Autodesk Inventor part; units mm, degrees
ref_plane "YZ Plane" through (0, 0, 0) normal (1, 0, 0) x (0, 1, 0)
ref_plane "XZ Plane" through (0, 0, 0) normal (0, 1, 0) x (-1, 0, 0)
ref_plane "XY Plane" through (0, 0, 0) normal (0, 0, 1) x (1, 0, 0)
sketch "Sketch2" plane through (0, 0, 0) normal (0, 0, 1) x (1, 0, 0)
  spline S0 degree 5 number of poles 204
  circle A0 centre (79.5137, 4.5678) radius 15.1135
  line L0 (79.5137, 4.5678) -> (79.5137, -15.4763) construction
  line L1 (79.5137, 4.5678) -> (209.6498, 4.5678) construction
  line L2 (319.6498, 0.0573) -> (219.6498, 0.0573) construction
  line L3 (219.6499, 18.7671) -> (219.6499, 18.7671) construction
  line L4 (28.0055, 4.5054) -> (28.0055, -2.4946)
  line L5 (19.6272, 1.0326) -> (319.6498, 0.0573) construction
  line L6 (49.7105, 14.4213) -> (55.6079, 14.4213)
  line L7 (49.7104, -8.4915) -> (55.6078, -8.4915)
  line L8 (28.0055, 4.5054) -> (49.7105, 14.4213)
  line L9 (28.0055, -2.4946) -> (49.7104, -8.4915)
  line L10 (55.6079, 14.4213) -> (55.6079, 20.8729)
  line L11 (55.6078, -8.4915) -> (55.6078, -14.1513)
  line L12 (108.6496, 16.3299) -> (108.6496, -7.1942)
  line L13 (110.8735, -9.1817) -> (193.8736, 0.1678)
  line L14 (195.6498, 2.1552) -> (195.6498, 6.9805)
  arc A1 (108.6496, -7.1942) -> (110.8735, -9.1817) centre (110.6496, -7.1942) ccw
  arc A2 (193.8736, 0.1678) -> (195.6498, 2.1552) centre (193.6498, 2.1552) ccw
  circle A3 centre (209.6498, 0.0573) radius 6.214
  line L15 (108.6496, 18.5678) -> (195.6498, 8.7678)
  circle A4 centre (100.6496, 18.3866) radius 2.5
  circle A5 centre (199.6498, 14.5256) radius 2.5
  spline S1 degree 4 poles (202.7347, 19.3724) (199.838, 19.7251) (195.7649, 20.2061) (190.5032, 20.7952) (184.0435, 21.4697) (179.3239, 21.937) (174.5933, 22.3806) (169.8562, 22.7962) (165.1183, 23.1863) (160.3828, 23.5463) (155.6566, 23.8767) (150.936, 24.1762) (146.2498, 24.4444) (141.5311, 24.676) (136.9019, 24.8782) (132.2312, 25.0296) (127.6189, 25.1375) (123.0371, 25.1983) (118.5028, 25.2125) (112.3622, 25.1677) (107.3995, 25.0507) (103.5849, 24.9119) (100.8865, 24.7866) knots 0 0 0 0 0 0.114234 0.16008 0.206003 0.251978 0.297982 0.343994 0.389991 0.435949 0.481846 0.527693 0.573431 0.619092 0.664656 0.710064 0.755333 0.800383 0.845191 0.889734 1 1 1 1 1
  line L16 (105.191, 21.4637) -> (195.6498, 15.3862)
  arc A6 (100.8865, 24.7866) -> (105.191, 21.4637) centre (100.0416, 19.2427) ccw
  arc A7 (195.6498, 15.3862) -> (202.7347, 19.3724) centre (200.4212, 15.1951) ccw
  point P0 (0, 0)
  point P1 (319.5771, 0.0748)
  point P2 (319.3573, 0.1272)
  point P3 (318.9916, 0.2136)
  point P4 (318.4804, 0.3362)
  point P5 (317.8238, 0.4909)
  point P6 (317.0222, 0.6802)
  point P7 (316.0769, 0.9024)
  point P8 (314.9885, 1.1569)
  point P9 (313.7582, 1.443)
  point P10 (312.3866, 1.7598)
  point P11 (310.8752, 2.1063)
  point P12 (309.2258, 2.4819)
  point P13 (307.4393, 2.8854)
  point P14 (305.5178, 3.3153)
  point P15 (303.4628, 3.7707)
  point P16 (301.2764, 4.2501)
  point P17 (298.9607, 4.7526)
  point P18 (296.5175, 5.2764)
  point P19 (293.9492, 5.8203)
  point P20 (291.2585, 6.3828)
  point P21 (288.4478, 6.9627)
  point P22 (285.5195, 7.5582)
  point P23 (282.4766, 8.1678)
  point P24 (279.3218, 8.79)
  point P25 (276.0584, 9.4236)
  point P26 (272.6891, 10.0668)
  point P27 (269.2175, 10.7178)
  point P28 (265.6469, 11.3757)
  point P29 (261.9803, 12.0381)
  point P30 (258.2219, 12.7041)
  point P31 (254.3747, 13.3722)
  point P32 (250.4426, 14.0403)
  point P33 (246.4295, 14.7072)
  point P34 (242.339, 15.3714)
  point P35 (238.1756, 16.0311)
  point P36 (233.9428, 16.6851)
  point P37 (229.6454, 17.3316)
  point P38 (225.2869, 17.9694)
  point P39 (220.8723, 18.5967)
  point P40 (216.4049, 19.2123)
  point P41 (211.8901, 19.8144)
  point P42 (207.332, 20.4015)
  point P43 (202.7347, 20.9724)
  point P44 (198.1034, 21.5256)
  point P45 (193.4423, 22.0596)
  point P46 (188.7563, 22.5726)
  point P47 (184.0499, 23.0637)
  point P48 (179.3279, 23.5314)
  point P49 (174.5948, 23.9745)
  point P50 (169.8554, 24.3909)
  point P51 (165.1148, 24.7803)
  point P52 (160.3775, 25.1406)
  point P53 (155.6479, 25.4709)
  point P54 (150.9316, 25.7703)
  point P55 (146.233, 26.0373)
  point P56 (141.557, 26.2707)
  point P57 (136.8821, 26.4681)
  point P58 (132.2209, 26.6211)
  point P59 (127.5964, 26.7282)
  point P60 (123.0133, 26.7888)
  point P61 (118.4727, 26.8026)
  point P62 (113.9902, 26.7693)
  point P63 (109.5601, 26.6886)
  point P64 (105.191, 26.5611)
  point P65 (100.8865, 26.3866)
  point P66 (96.6524, 26.1647)
  point P67 (92.4927, 25.8975)
  point P68 (88.412, 25.5858)
  point P69 (84.409, 25.3061)
  point P70 (80.8803, 24.9766)
  point P71 (76.6761, 24.4558)
  point P72 (72.9631, 23.8932)
  point P73 (69.3402, 23.3612)
  point P74 (65.8208, 22.7938)
  point P75 (62.4086, 22.1884)
  point P76 (59.1071, 21.5462)
  point P77 (52.8493, 20.1606)
  point P78 (49.7107, 19.4213)
  point P79 (47.0737, 18.6508)
  point P80 (44.3741, 17.8542)
  point P81 (41.8033, 17.0323)
  point P82 (39.3638, 16.1875)
  point P83 (37.0582, 15.3214)
  point P84 (34.8883, 14.4364)
  point P85 (32.8567, 13.534)
  point P86 (30.9649, 12.6166)
  point P87 (29.2144, 11.686)
  point P88 (27.607, 10.7437)
  point P89 (26.1442, 9.7921)
  point P90 (24.8269, 8.8324)
  point P91 (23.6566, 7.8664)
  point P92 (22.6337, 6.8952)
  point P93 (21.7592, 5.9208)
  point P94 (21.0335, 4.944)
  point P95 (20.4573, 3.966)
  point P96 (20.031, 2.9874)
  point P97 (19.7541, 2.0097)
  point P98 (19.6496, 0.0598)
  point P99 (19.8207, -0.9032)
  point P100 (20.1378, -1.8356)
  point P101 (20.6004, -2.7401)
  point P102 (21.2081, -3.6158)
  point P103 (21.9599, -4.4627)
  point P104 (22.8545, -5.2806)
  point P105 (23.891, -6.069)
  point P106 (25.0682, -6.8277)
  point P107 (26.3845, -7.5561)
  point P108 (27.8383, -8.2539)
  point P109 (29.4283, -8.9211)
  point P110 (31.1522, -9.5571)
  point P111 (33.0086, -10.1613)
  point P112 (34.9949, -10.734)
  point P113 (37.1093, -11.2746)
  point P114 (39.3497, -11.7828)
  point P115 (41.7134, -12.2586)
  point P116 (44.1979, -12.702)
  point P117 (46.8014, -13.1127)
  point P118 (49.7105, -13.4915)
  point P119 (52.3532, -13.8357)
  point P120 (58.3469, -14.4294)
  point P121 (61.5023, -14.678)
  point P122 (64.7591, -14.8953)
  point P123 (68.1149, -15.0813)
  point P124 (71.5661, -15.237)
  point P125 (75.1094, -15.3627)
  point P126 (78.7418, -15.4596)
  point P127 (82.46, -15.528)
  point P128 (86.2607, -15.5691)
  point P129 (90.14, -15.5838)
  point P130 (94.0946, -15.5733)
  point P131 (98.1212, -15.5388)
  point P132 (102.2159, -15.4812)
  point P133 (106.3751, -15.4023)
  point P134 (110.5952, -15.303)
  point P135 (114.872, -15.1845)
  point P136 (119.2022, -15.0489)
  point P137 (123.5813, -14.8971)
  point P138 (128.006, -14.7306)
  point P139 (132.4718, -14.5509)
  point P140 (136.9748, -14.3598)
  point P141 (141.5285, -14.1576)
  point P142 (146.1365, -13.9383)
  point P143 (150.7679, -13.7022)
  point P144 (155.4191, -13.4499)
  point P145 (160.0853, -13.1829)
  point P146 (164.7617, -12.9024)
  point P147 (169.4444, -12.6099)
  point P148 (174.1283, -12.306)
  point P149 (178.8092, -11.9925)
  point P150 (183.4823, -11.67)
  point P151 (188.1434, -11.34)
  point P152 (192.7877, -11.0037)
  point P153 (197.4107, -10.6614)
  point P154 (202.0079, -10.3149)
  point P155 (206.5747, -9.9645)
  point P156 (211.1069, -9.6117)
  point P157 (215.5999, -9.2568)
  point P158 (220.0489, -8.9007)
  point P159 (224.4503, -8.5446)
  point P160 (228.7987, -8.1885)
  point P161 (233.0906, -7.8339)
  point P162 (237.3214, -7.4808)
  point P163 (241.4866, -7.1298)
  point P164 (245.5828, -6.7821)
  point P165 (249.6052, -6.4377)
  point P166 (253.5502, -6.0972)
  point P167 (257.4136, -5.7612)
  point P168 (261.1915, -5.4303)
  point P169 (264.88, -5.1051)
  point P170 (268.4758, -4.7856)
  point P171 (271.9747, -4.4724)
  point P172 (275.3734, -4.1661)
  point P173 (278.6686, -3.867)
  point P174 (281.8564, -3.5757)
  point P175 (284.9344, -3.2925)
  point P176 (287.8984, -3.018)
  point P177 (290.7463, -2.7525)
  point P178 (293.4745, -2.4963)
  point P179 (296.0806, -2.2503)
  point P180 (298.5616, -2.0142)
  point P181 (300.9151, -1.7892)
  point P182 (303.1387, -1.575)
  point P183 (305.23, -1.3728)
  point P184 (307.1866, -1.1823)
  point P185 (309.007, -1.0041)
  point P186 (310.6885, -0.8385)
  point P187 (312.2302, -0.6861)
  point P188 (313.6297, -0.5471)
  point P189 (314.8861, -0.4221)
  point P190 (315.9976, -0.3107)
  point P191 (316.9636, -0.214)
  point P192 (317.7826, -0.1311)
  point P193 (318.4538, -0.0643)
  point P194 (318.9765, -0.0102)
  point P195 (319.3503, 0.027)
  point P196 (319.5743, 0.0497)
  point P197 (28.0055, 1.0054)
  point P198 (108.6496, -9.4322)
  point P199 (195.6498, 0.3678)
  dimension "d37" = 30.227
  dimension "d2" = 300.0001
  dimension "d19" = 110
  dimension "d22" = 100
  dimension "d23" = 7
  dimension "d24" = 5
  dimension "d25" = 5
  dimension "d30" = 28
  dimension "d31" = 8.4
  dimension "d33" = 14
  dimension "d39" = 59.8865
  dimension "d42" = 12.428
  dimension "d43" = 5
  dimension "d44" = 5
  dimension "d49" = 1.6
  dimension "d50" = 1.6
  dimension "d51" = 1.6
  dimension "d52" = 1.6
  dimension "d53" = 1.6
  dimension "d54" = 1.6
  dimension "d55" = 1.6
  dimension "d56" = 1.6
  dimension "d57" = 1.6
  dimension "d58" = 1.6
  dimension "d59" = 1.6
  dimension "d60" = 1.6
  dimension "d61" = 1.6
  dimension "d62" = 1.6
  dimension "d63" = 1.6
  dimension "d64" = 1.6
  dimension "d65" = 1.6
  dimension "d66" = 1.6
  dimension "d67" = 1.6
  dimension "d68" = 1.6
  dimension "d69" = 1.6
  dimension "d70" = 1.6
  dimension "d72" = 1.6
  dimension "d75" = 4
  dimension "d76" = 7
  dimension "d90" = 8
  dimension "d91" = 8
extrude "Extrusion8" add sketch "Sketch2" along normal blind 54 contours A7 L16 A6 S1
sketch "Sketch3" plane through (195.6498, 15.3862, 0) normal (-0.067, -0.9978, 0) x (0.9978, -0.067, 0)
  line L0 (-0.0017, 49) -> (-0.0017, 5)
  line L1 (-0.0017, 5) -> (-22.7277, 26.2297)
  line L2 (-22.7277, 26.2297) -> (-0.0017, 49)
  line L3 (-67.7277, 27.0011) -> (-45.2277, 49.0011)
  line L4 (-45.2277, 49.0011) -> (-45.2277, 5.0011)
  line L5 (-45.2277, 5.0011) -> (-67.7277, 27.0011)
  line L6 (-45.2277, 49.0011) -> (-22.7277, 26.2297)
  line L7 (-45.2277, 5.0011) -> (-22.7277, 26.2297)
  line L8 (9.5487, 54) -> (0, 54)
  line L9 (9.5487, 0) -> (0, 0)
  line L10 (-90.2837, 49) -> (-90.1718, 5)
  line L11 (-90.1718, 5) -> (-67.7277, 27.0011)
  line L12 (-90.2837, 49) -> (-67.7277, 27.0011)
  line L13 (-90.0437, 54) -> (-101.2596, 54)
  line L14 (-90.0437, 0) -> (-101.2596, 0)
  line L15 (-90.2837, 49) -> (-0.0017, 49)
  line L16 (-0.0017, 5) -> (-90.1718, 5)
  line L17 (-86.7403, 49) -> (-45.0868, 9.6057)
  line L18 (-86.7403, 5) -> (-45.2277, 44.1668)
  line L19 (-45.2277, 44.1668) -> (-5.985, 5)
  line L20 (-5.985, 49) -> (-45.2277, 9.739)
  line L21 (-47.5072, 5) -> (-47.5072, 49)
  line L22 (-42.3779, 49) -> (-42.3779, 5)
  point P0 (-194.1783, 0)
  point P1 (-90.6627, 0)
  point P2 (-45.2277, 27.0011)
  point P3 (6.8018, 54)
  point P4 (6.8018, 0)
  point P5 (-95.1802, 54)
  point P6 (-90.6627, 54)
  point P7 (-95.1802, 0)
  point P8 (-28.0012, 26.9736)
  point P9 (-63.4507, 26.9736)
  point P10 (-25.7189, 29.2569)
  point P11 (-45.2266, 49)
  point P12 (-65.6391, 29.0433)
  point P13 (-45.2288, 49)
  point P14 (-25.0554, 24.0335)
  point P15 (-65.6131, 24.9334)
  point P16 (-42.3779, 7.6899)
  point P17 (-42.3779, 41.3225)
  point P18 (-42.3779, 12.5902)
  point P19 (-42.3779, 46.1169)
  point P20 (-47.5072, 46.7723)
  point P21 (-47.5072, 7.23)
  point P22 (-47.5072, 11.8949)
  point P23 (-47.5072, 42.0161)
  dimension "d81" = 22.5
  dimension "d82" = 22.5
  dimension "d83" = 5
  dimension "d84" = 5
  dimension "d85" = 22.5
  dimension "d86" = 5
  dimension "d87" = 5
extrude "Extrusion9" cut sketch "Sketch3" against normal blind 10 contours L0 L1 L2 | L20 L6 L22 L15 | L16 L22 L7 L19 | L20 L22 L19 | L3 L17 L15 L21 | L21 L16 L18 L5 | L21 L17 L18 | L11 L10 L12
properties part number "2414 basic aerofoil" material "Plywood, Finish"
The model under review builds one solid part; all positions refer to its coordinate system, in mm. A direction names the side the tool comes from. Give positions to 0.01 mm unless a question says otherwise; leave off trailing zeros. Answer in a Markdown table with one row per item. Add a question column.
1. Insertion check: P1, Ø3, axis at x = 194, y = 12, coming from the -Z side; P2, Ø1.5, axis at y = 18, z = 31.5, coming from the -X side. Each pin has a flat end and moves straight along its axis. Give the tip position at first contact, or say it passes through.
2. We need section A-A on z = 37. State how many separate pieces and enclosed holes the cut face has, then the cut area to 3 significant figures.
3. Wall thickness on line 1 along Z through (x, y) = (181.5, 20.5); line 2 along X through (y, z) = (16.5, 28); line 3 along X through (y, z) = (16.25, 11): over which ranges is each line inside the solid? List them lowest first. Write a range as [from, to].
4. Draft analysis for pull direction Z (two halves, no side actions). For faces 3 (the flat face through (161.753, 20.522, 37.805)), 4 (the flat face through (153.56, 21.07, 27.16)), 5 (the flat face through (149, 21, 54)), 6 (the cylindrical face through (202.885, 11.105, 26.622)), state which applies: +Z half, -Z half, draft (parallel to the pull), parting line (faces both ways), or undercut.
5. Tool access review of faces 1 (the flat face through (153.56, 21.07, 47.58)), 2 (the flat face through (195.807, 17.746, 27.308)): name each direction out of +Z, -Z, +X, -X, +Y, -Y from which nothing blocks a thin tool from reaching the whole face with its end or side.
Ans:
| question | item | result |
|---|---|---|
| 1 | P1 | passes through |
| 1 | P2 | stops at x = 94.46 |
| 2 | separate pieces | 7 |
| 2 | enclosed holes | 2 |
| 2 | area | 275 mm^2 |
| 3 | line 1 | z = [0, 5], [13.46, 18.51], [34.51, 40.52], [49, 54] |
| 3 | line 2 | x = [95.15, 99.01], [102.29, 104.93], [195.72, 198.12], [201.18, 205.01] |
| 3 | line 3 | x = [95.3, 99.35], [101.95, 104.78], [183.68, 189.27], [195.71, 197.84], [201.46, 205.08] |
| 4 | face 3 | undercut |
| 4 | face 4 | undercut |
| 4 | face 5 | +Z half |
| 4 | face 6 | draft |
| 5 | face 1 | -Y |
| 5 | face 2 | +Y |
